Verification items for this drawing (mm, ordinates from the low corner). A direction names the side the tool comes from. Coordinates: 2 decimals unless noted, no trailing zeros. Order: outer loops, then holes, each group sorted by start corner. A loop starts at its lowest first (then second) coordinate and runs counter-clockwise, first axis right, second up. Notation, with made-up numbers: M 0.25,50.25 L 11.25,50.25 A18 cw 11.25,55.25 Z; hole C 86.25,26.5 d9. An arc over 180 degrees is marked long. One line per item, written item: value. Start each with the question number.
1) Access from +Z, -Z, +X, -X, +Y, -Y to the whole of each face (thin tool, end or side, straight path). Record for the marked faces 1, 2 and 3.
2) Sectioned sample at B-B, the plane x = 30. Enter the section's corners in (y, z), then the cut area to 3 significant figures.
3) Sectioned sample at D-D, the plane y = 17.5. Enter the section's corners in (x, z), then the cut area to 3 significant figures.
4) Sectioned sample at A-A, the plane y = 1.75. State how many separate pieces and enclosed holes the cut face has, then the cut area to 3 significant figures.
5) Sectioned sample at C-C, the plane z = 19.25. Enter the section's corners in (x, y).
6) Thickness scan on L1, parallel to Z at x = 22.5, y = 8.25; L2, parallel to Z at x = 8, y = 2; L3, parallel to Y at x = 33.5, z = 19. Record the ranges inside material, lowest first. Write a range as from..to.
7) Draft check along Y on the marked faces 4, 5 and 6. Enter one of: pulls with the +Y half, pulls with the -Y half, needs draft (parallel to the pull), parting line crosses it, or undercut.
8) Go/stop test with flat-tipped pins: P1, Ø4, axis at y = 7.5, z = 18.5, coming from the -X side; P2, Ø4, axis at y = 12.5, z = 18.5, coming from the +X side; P3, Ø4, axis at y = 18.5, z = 9.5, coming from the -X side. Record where each tip stops, or that it passes through.
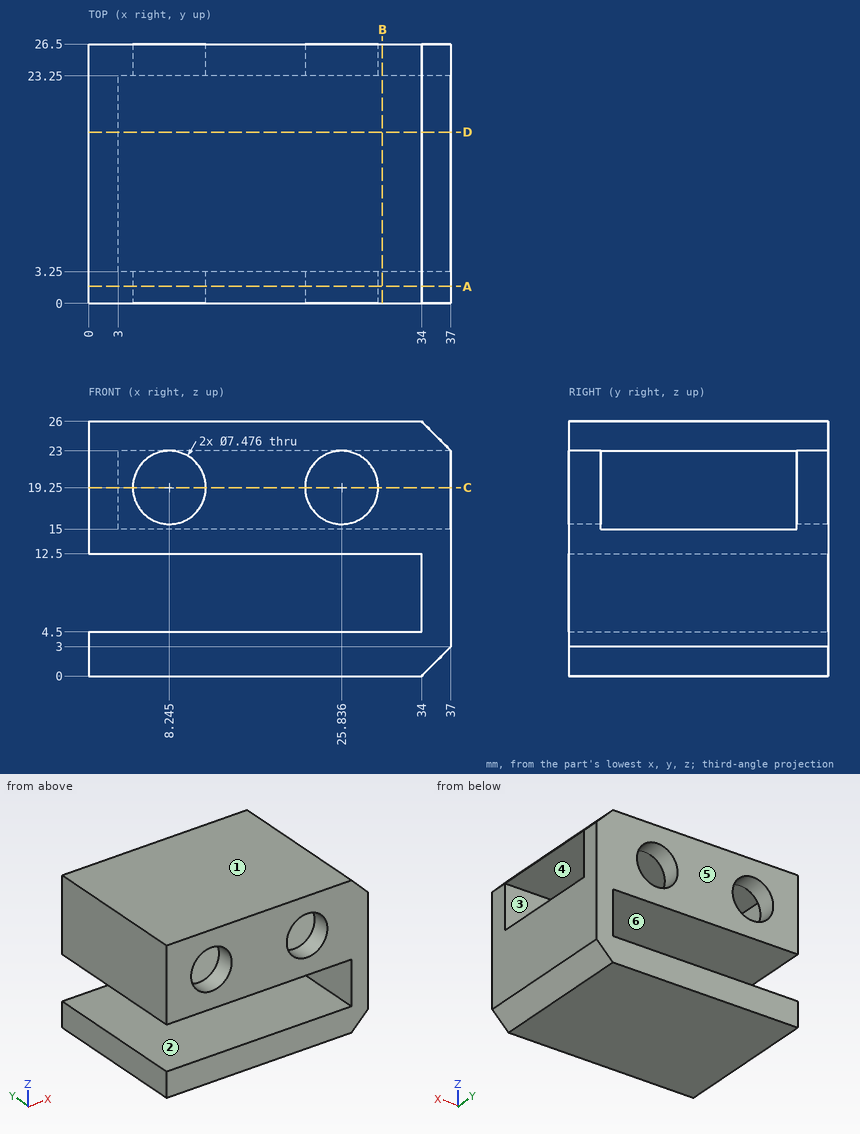
Final values:
1. face 1: +Z, +X, -X, +Y, -Y
1. face 2: -X, +Y, -Y
1. face 3: +X
2. outline: M 0,0 L 26.5,0 L 26.5,4.5 L 0,4.5 Z; M 0,12.5 L 26.5,12.5 L 26.5,26 L 0,26 Z; hole M 3.25,15 L 23.25,15 L 23.25,23 L 3.25,23 Z
2. area: 317 mm^2
3. outline: M 0,0 L 34,0 L 37,3 L 37,15 L 3,15 L 3,23 L 37,23 L 34,26 L 0,26 L 0,12.5 L 34,12.5 L 34,4.5 L 0,4.5 Z
3. area: 409 mm^2
4. separate pieces: 1
4. enclosed holes: 2
4. area: 593 mm^2
5. outline: M 0,0 L 4.51,0 L 4.51,3.25 L 3,3.25 L 3,23.25 L 4.51,23.25 L 4.51,26.5 L 0,26.5 Z; M 11.98,0 L 22.1,0 L 22.1,3.25 L 11.98,3.25 Z; M 11.98,23.25 L 22.1,23.25 L 22.1,26.5 L 11.98,26.5 Z; M 29.57,0 L 37,0 L 37,3.25 L 29.57,3.25 Z; M 29.57,23.25 L 37,23.25 L 37,26.5 L 29.57,26.5 Z
6. L1: z = 0..4.5, 12.5..15, 23..26
6. L2: z = 0..4.5, 12.5..15.52, 22.98..26
6. L3: y = 0..3.25, 23.25..26.5
7. face 4: undercut
7. face 5: pulls with the +Y half
7. face 6: needs draft
8. P1: stops at x = 0
8. P2: stops at x = 3
8. P3: stops at x = 34
